For this review, take the finished solid that the model builds, in its own axes (mm). A direction names the side the tool comes from. Round coordinates to 2 decimals unless told otherwise and drop trailing zeros. Write each loop counter-clockwise with the first axis right and the second up, starting at its lowest first coordinate (ties: lowest second). Pieces come first, ordered by that corner, then holes. Notation, with made-up numbers: M 23.25,60.25 L 47.25,60.25 A21 ccw 47.25,69.25 Z; hole C -37,-36 d3. An arc over 180 degrees is marked long. Use one line per item in the form item = value. Start each with the question number.
Item 1: For faces 1 (the flat face through (0.1, 20, -8.5)), 2 (the cylindrical face through (0, 1, 6)), 3 (the flat face through (0, 5, -10)), 4 (the flat face through (-4, 2, 1)), 5 (the flat face through (-9, 19, -6)), list the 3-axis set-ups (+Z, -Z, +X, -X, +Y, -Y) from which the entire face can be reached by the end or side of a thin tool; tool diameter is ignored.
Item 2: Add section C-C (z = -1.75). State the section outline as (x, y) points.
Item 3: For line 1 (X direction, y = 2.25, z = 4.5); line 2 (Z direction, x = 5.5, y = 9.5); line 3 (Y direction, x = -3.75, z = 5.5), list the stretches that pass through material, from the lowest coordinate up. Write a range as [from, to].
Item 4: For P1, Ø8, axis at x = -2, y = 9.5, coming from the +Z side; P2, Ø1.6, axis at x = -9, y = 18.5, coming from the +Z side; P3, Ø2, axis at x = -1.5, y = 8, coming from the -Z side, all flat-tipped, find the tip position at first contact; note any pin that passes through.
Item 5: Add section A-A (x = 0). State the section outline as (y, z) points, and give its area (3 significant figures).
Item 6: Draft analysis for pull direction Y (two halves, no side actions). For faces 6 (the flat face through (9, 11, 1)), 7 (the flat face through (3, 1, 1)), 8 (the flat face through (-3, 11, -9)), state which applies: released by +Y, released by -Y, zero draft, split by the parting line, or undercut.
Item 7: Add section D-D (y = 17.5). State the section outline as (x, z) points, and give its area (3 significant figures).
Item 8: Add section B-B (y = 10.5). State the section outline as (x, z) points, and give its area (3 significant figures).
from build123d import *

# Parameters (mm, degrees)
SKETCH2_W               = 20
SKETCH2_H               = 20
BOSS_EXTRUDE1_DEPTH     = 2
SKETCH4_W               = 20
SKETCH4_H               = 20
BOSS_EXTRUDE2_DEPTH     = 2
BOSS_EXTRUDE3_DEPTH     = 2
CUT_EXTRUDE1_DEPTH      = 23.891046285
CUT_EXTRUDE1_DEPTH_BACK = 23.891046285
CUT_EXTRUDE2_DEPTH      = 29.705400189
CUT_EXTRUDE2_DEPTH_BACK = 29.705400189


with BuildPart() as part:
    # Sketch2 → Boss-Extrude1 (new body)
    with BuildSketch(Plane(origin=(0, 0, 0), x_dir=(1, 0, 0), z_dir=(0, 1, 0))):
        Rectangle(SKETCH2_W, SKETCH2_H)
    extrude(amount=BOSS_EXTRUDE1_DEPTH)

    # Sketch4 → Boss-Extrude2 (add)
    with BuildSketch(Plane(origin=(0, 0, -10), x_dir=(-1, 0, 0), z_dir=(0, 0, -1))):
        with Locations((0, 10)):
            Rectangle(SKETCH4_W, SKETCH4_H)
    extrude(amount=-BOSS_EXTRUDE2_DEPTH)

    # Sketch5 → Boss-Extrude3 (add)
    with BuildSketch(Plane.ZY.offset(10)):
        Polygon((-6, 18), (8, 4), (10, 4), (10, 2), (-8, 2), (-8, 20), (-6, 20), align=None)
    boss_extrude3 = extrude(amount=-BOSS_EXTRUDE3_DEPTH)

    # Mirror1: Boss-Extrude3 across plane
    add(boss_extrude3.mirror(Plane(origin=(0, 0, 0), x_dir=(0, 0, 1), z_dir=(1, 0, 0))))

    # Sketch6 → Cut-Extrude1 (cut, two sides: drawn at the far end of the back side and taken through both)
    with BuildSketch(Plane(origin=(0, 2, 0), x_dir=(1, 0, 0), z_dir=(0, 1, 0)).offset(-CUT_EXTRUDE1_DEPTH_BACK)):
        with BuildLine():
            Line((3, 1), (3, -3))
            ThreePointArc((3, -3), (0, -6), (-3, -3))
            Line((-3, -3), (-3, 1))
            ThreePointArc((-3, 1), (0, 4), (3, 1))
        make_face()
    extrude(amount=CUT_EXTRUDE1_DEPTH + CUT_EXTRUDE1_DEPTH_BACK, mode=Mode.SUBTRACT)

    # Sketch7 → Cut-Extrude2 (cut, two sides: drawn at the far end of the back side and taken through both)
    with BuildSketch(Plane.XY.offset(-8).offset(-CUT_EXTRUDE2_DEPTH_BACK)):
        with BuildLine():
            Line((3, 13), (3, 9))
            ThreePointArc((3, 9), (0, 6), (-3, 9))
            Line((-3, 9), (-3, 13))
            ThreePointArc((-3, 13), (0, 16), (3, 13))
        make_face()
    extrude(amount=CUT_EXTRUDE2_DEPTH + CUT_EXTRUDE2_DEPTH_BACK, mode=Mode.SUBTRACT)


solid = part.part
Calculated:
q1.face_1 = +Z, -Z, +X, -X, +Y
q1.face_2 = +Y, -Y
q1.face_3 = -Z, +X, -X, +Y, -Y
q1.face_4 = +Z, +Y
q1.face_5 = +Z, +X, -X, +Y
q2.outline = M -10,0 L -2.9,0 L -2.9,2 L -8,2 L -8,13.75 L -10,13.75 Z; M 2.9,0 L 10,0 L 10,13.75 L 8,13.75 L 8,2 L 2.9,2 Z
q3.line_1 = [-10, -8], [8, 10]
q3.line_2 = [-10, -8]
q3.line_3 = [0, 2]
q4.P1 = -8
q4.P2 = -5.7
q4.P3 = through
q5.outline = M 0,-10 L 6,-10 L 6,-8 L 2,-8 L 2,-4 L 0,-4 Z; M 0,6 L 2,6 L 2,10 L 0,10 Z; M 16,-10 L 20,-10 L 20,-8 L 16,-8 Z
q5.area = 36.0 mm^2
q6.face_6 = released by +Y
q6.face_7 = zero draft
q6.face_8 = undercut
q7.outline = M -10,-10 L 10,-10 L 10,-5.5 L 8,-5.5 L 8,-8 L -8,-8 L -8,-5.5 L -10,-5.5 Z
q7.area = 50.0 mm^2
q8.outline = M -10,-10 L -3,-10 L -3,-8 L -8,-8 L -8,1.5 L -10,1.5 Z; M 3,-10 L 10,-10 L 10,1.5 L 8,1.5 L 8,-8 L 3,-8 Z
q8.area = 66.0 mm^2
